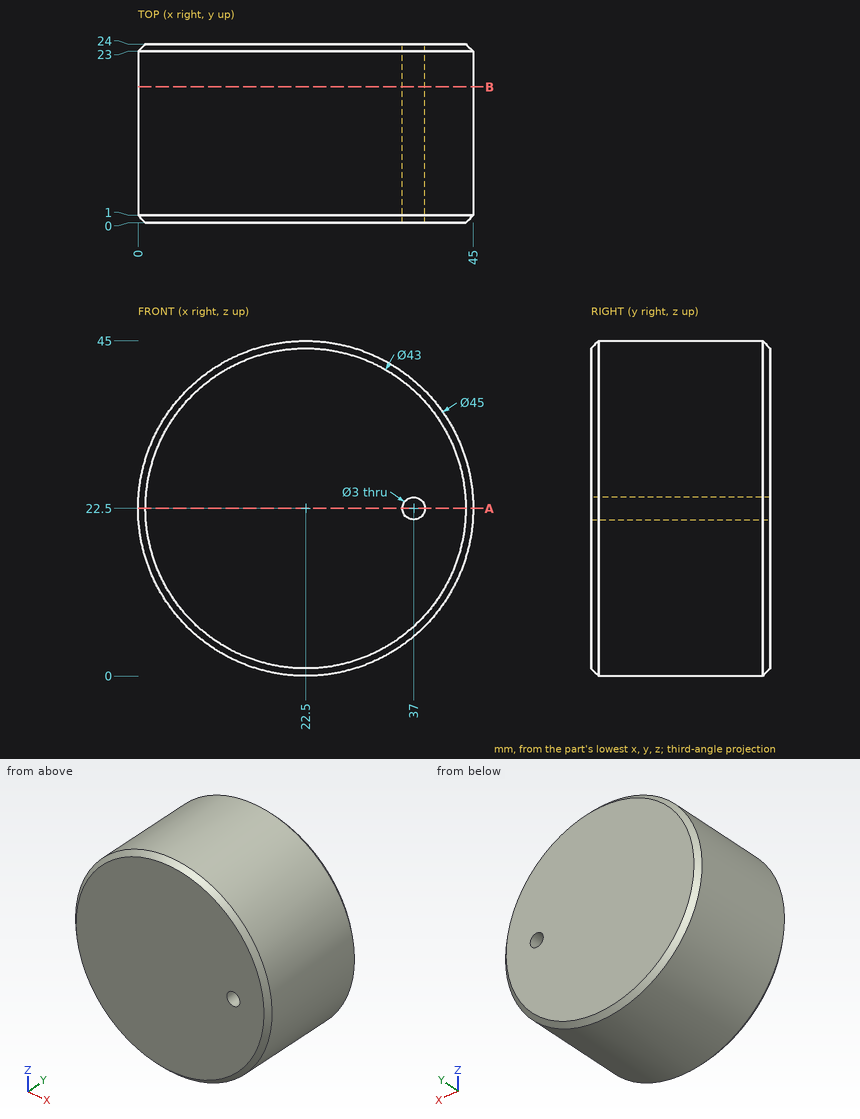
Study the drawing (mm; zero at the part's minimum x, y, z) and answer. Coordinates: 2 decimals unless noted, no trailing zeros. Loops run counter-clockwise (first coordinate to the right, second up) from the corner with the lowest first, then second, coordinate; pieces in that order, holes last. Notation, with made-up numbers: (20.25, 17.25) -> (60.25, 17.25) arc R25 cw to (60.25, 38.25) -> close; hole circle Ø6 at (68, 64.25). An arc over 180 degrees is marked (long way). Write each question's results on one line, items separated by ' | '. Start each with the question number.
1) Consider line 1 along X through (y, z) = (14, 22.5); line 2 along Z through (x, y) = (22, 4); line 3 along Z through (x, y) = (36, 9.5). Determine where each line is inside the solid, lowest interval first.
2) Flat-ended cylindrical pins translate along their axes: P1, Ø2, axis at x = 34, y = 21, coming from the -Z side; P2, Ø2, axis at y = 10, z = 12, coming from the +X side; P3, Ø3, axis at y = 5.5, z = 26.5, coming from the -X side. Find the tip coordinate at first contact, or state that the pin passes through.
3) Find section A-A on z = 22.5. Determine the outline of the cut face in (x, y).
4) Find section B-B on y = 18.25. Determine the outline of the cut face in (x, z), then the cut area to 3 significant figures.
Response values:
1) line 1: x = 0 to 35.5, 38.5 to 45 | line 2: z = 0.01 to 44.99 | line 3: z = 4.5 to 21.38, 23.62 to 40.5
2) P1: stops at z = 2.6 | P2: stops at x = 42.9 | P3: stops at x = 0.14
3) outline: (0, 1) -> (1, 0) -> (35.5, 0) -> (35.5, 24) -> (1, 24) -> (0, 23) -> close; (38.5, 0) -> (44, 0) -> (45, 1) -> (45, 23) -> (44, 24) -> (38.5, 24) -> close
4) outline: circle Ø45 at (22.5, 22.5); hole circle Ø3 at (37, 22.5) | area: 1,580 mm^2
